from build123d import *

# Parameters (mm, degrees)
SKETCH1_R           = 3.175
SKETCH1_R_2         = 2.38125
BOSS_EXTRUDE1_DEPTH = 1.5875
SKETCH2_R           = 5.08
SKETCH2_R_2         = 2.38125
BOSS_EXTRUDE2_DEPTH = 1.016
FILLET1_R           = 0.762


with BuildPart() as part:
    # Sketch1 → Boss-Extrude1 (new body)
    with BuildSketch(Plane(origin=(0, 0, 0), x_dir=(1, 0, 0), z_dir=(0, 1, 0))):
        Circle(SKETCH1_R)
        Circle(SKETCH1_R_2, mode=Mode.SUBTRACT)
    extrude(amount=BOSS_EXTRUDE1_DEPTH)

    # Sketch2 → Boss-Extrude2 (add)
    with BuildSketch(Plane(origin=(0, 1.5875, 0), x_dir=(1, 0, 0), z_dir=(0, 1, 0))):
        Circle(SKETCH2_R)
        Circle(SKETCH2_R_2, mode=Mode.SUBTRACT)
    extrude(amount=BOSS_EXTRUDE2_DEPTH)

    # Fillet1
    fillet1_edges = [part.edges().sort_by_distance(p)[0] for p in [
        (-2.38125, 2.6035, 0),
        (-5.08, 2.6035, 0),
    ]]
    fillet(fillet1_edges, radius=FILLET1_R)


solid = part.part
Part model, mm, in its own coordinate system. Coordinates: 2 decimals unless noted, no trailing zeros. Order: outer loops, then holes, each group sorted by start corner. A loop starts at its lowest first (then second) coordinate and runs counter-clockwise, first axis right, second up. Notation, with made-up numbers: M 79,29.25 L 100,29.25 A13 ccw 100,36.25 Z; hole C -40,65.5 d9. An arc over 180 degrees is marked long. Use a Markdown table: item, result.
(1) Pull direction X, two halves, no side cores. Call faces 1 (the cylindrical face through (-1.89, 0.91, 1.45)), 2 (the flat face through (3.3, 1.588, 1.1)), 3 (the cylindrical face through (-0.69, 0.78, 3.1)): released by +X, released by -X, zero draft, split by the parting line, or undercut.
A:
| item | result |
|---|---|
| face 1 | undercut |
| face 2 | zero draft |
| face 3 | split by the parting line |
(2) Probe L1, parallel to X at y = 0.65, z = 0 (3 decimals); L2, parallel to Y at x = -3.25, z = 0. List the from-to ranges inside material, lowest first.
A:
| item | result |
|---|---|
| L1 | x = -3.175 to -2.381, 2.381 to 3.175 |
| L2 | y = 1.59 to 2.6 |
(3) Cut at D-D on y = 2.45. Write the cut outline in (x, z).
A:
| item | result |
|---|---|
| outline | C 0,0 d9.55; hole C 0,0 d5.37 |
(4) Flat gauge pins, fed straight in: pin 1 (3 mm diameter, centred on x = 0, z = 2, fed in from -Y); pin 2 (3 mm diameter, centred on x = 0, z = 0, fed in from +Y); pin 3 (1.5 mm diameter, centred on x = -1, y = 0.5, fed in from +Z). Where does each tip first touch, or does it go through?
A:
| item | result |
|---|---|
| pin 1 | stops at y = 0 |
| pin 2 | passes through |
| pin 3 | stops at z = 3.17 |
